Source: CAD feature listing. Evaluate the final solid. Frame: model axes, mm. A direction names the side the tool comes from. Give positions to 0.01 mm unless a question says otherwise; leave off trailing zeros. Loops run counter-clockwise (first coordinate to the right, second up) from the corner with the lowest first, then second, coordinate; pieces in that order, holes last. Notation, with made-up numbers: M 5,-1 L 64,-1 A6 ccw 64,6 Z; hole C 30,-17 d5. An arc over 180 degrees is marked long. Answer in a Markdown table with one row per item.
```python
from build123d import *

# Parameters (mm, degrees)
SKETCH_1_W          = 9
SKETCH_1_H          = 9
EXTRUDE_1_DEPTH     = 81.5
SKETCH_2_W          = 7
SKETCH_2_H          = 7
CUT_EXTRUDE_1_DEPTH = 101.5
SKETCH_3_R          = 3
SKETCH_3_R_2        = 1.5
CUT_EXTRUDE_2_DEPTH = 111.5
SKETCH_4_R          = 3
CUT_EXTRUDE_3_DEPTH = 1


with BuildPart() as part:
    # ｽｹｯﾁ1 → ﾎﾞｽ - 押し出し1 (new body)
    with BuildSketch(Plane.XY):
        Rectangle(SKETCH_1_W, SKETCH_1_H)
    extrude(amount=EXTRUDE_1_DEPTH)

    # ｽｹｯﾁ2 → ｶｯﾄ - 押し出し1 (cut)
    with BuildSketch(Plane.XY.offset(81.5)):
        Rectangle(SKETCH_2_W, SKETCH_2_H)
    extrude(amount=-CUT_EXTRUDE_1_DEPTH, mode=Mode.SUBTRACT)

    # ｽｹｯﾁ3 → ｶｯﾄ - 押し出し2 (cut)
    with BuildSketch(Plane(origin=(0, 4.5, 0), x_dir=(1, 0, 0), z_dir=(0, 1, 0))):
        with Locations((0, -5)):
            Circle(SKETCH_3_R)
        with Locations((0, -11.5)):
            Circle(SKETCH_3_R_2)
        with Locations((0, -76.5)):
            Circle(SKETCH_3_R_2)
    extrude(amount=-CUT_EXTRUDE_2_DEPTH, mode=Mode.SUBTRACT)

    # ｽｹｯﾁ4 → ｶｯﾄ - 押し出し3 (cut)
    with BuildSketch(Plane(origin=(0, 4.5, 0), x_dir=(1, 0, 0), z_dir=(0, 1, 0))):
        with Locations((0, -76.5)):
            Circle(SKETCH_4_R)
    extrude(amount=-CUT_EXTRUDE_3_DEPTH, mode=Mode.SUBTRACT)


solid = part.part
```
Q1. Section query D-D (z = 21). Output: boundary loops of the cut face in (x, y).
Values follow:
| item | result |
|---|---|
| outline | M -4.5,-4.5 L 4.5,-4.5 L 4.5,4.5 L -4.5,4.5 Z; hole M -3.5,-3.5 L 3.5,-3.5 L 3.5,3.5 L -3.5,3.5 Z |
Q2. Ray query, probe 1 along Z at (x, y) = (0, -4.05); probe 2 along X at (y, z) = (-4.1, 5); probe 3 along X at (y, z) = (2.5, 29.5). Return the intervals inside material, ascending. Write a range as from..to.
Values follow:
| item | result |
|---|---|
| probe 1 | 0..2, 8..10, 13..75, 78..81.5 |
| probe 2 | -4.5..-3, 3..4.5 |
| probe 3 | -4.5..-3.5, 3.5..4.5 |
Q3. Contact query for a flat-ended pin moving along its axis: pin 1 Ø1.8 at (x, z) = (0, 11.5) entering from -Y. Output: stop coordinate, or through.
Values follow:
| item | result |
|---|---|
| pin 1 | through |
Q4. Section query A-A (x = 0). Give the number of separate pieces and of enclosed holes in the cut face, plus the area to 3 significant figures.
Values follow:
| item | result |
|---|---|
| separate pieces | 8 |
| enclosed holes | 0 |
| area | 136 mm^2 |
Q5. Mould query, pull axis Z, two halves, no side actions, for faces 1 (the cylindrical face through (0, -4, 13)), 2 (the flat face through (-4, 0, 81.5)), 3 (the flat face through (0, 3.5, 41)). Classes: +Z half, -Z half, draft (parallel to the pull), parting line (faces both ways), or undercut.
Values follow:
| item | result |
|---|---|
| face 1 | undercut |
| face 2 | +Z half |
| face 3 | draft |
Q6. Section query B-B (z = 76.5). Output: boundary loops of the cut face in (x, y), plus the area to 3 significant figures.
Values follow:
| item | result |
|---|---|
| outline | M -4.5,-4.5 L -1.5,-4.5 L -1.5,-3.5 L -3.5,-3.5 L -3.5,3.5 L -3,3.5 L -3,4.5 L -4.5,4.5 Z; M 1.5,-4.5 L 4.5,-4.5 L 4.5,4.5 L 3,4.5 L 3,3.5 L 3.5,3.5 L 3.5,-3.5 L 1.5,-3.5 Z |
| area | 23.0 mm^2 |
Q7. Section query C-C (y = -2.5). Output: boundary loops of the cut face in (x, z), plus the area to 3 significant figures.
Values follow:
| item | result |
|---|---|
| outline | M -4.5,0 L -3.5,0 L -3.5,81.5 L -4.5,81.5 Z; M 3.5,0 L 4.5,0 L 4.5,81.5 L 3.5,81.5 Z |
| area | 163 mm^2 |
Q8. Reachability of faces 4 (the cylindrical face through (-0.65, 4.01, 79.43)), 5 (the cylindrical face through (0.806, -3.993, 75.235)), 6 (the flat face through (3.5, 0, 41)) from +Z, -Z, +X, -X, +Y, -Y: full face, straight path, thin tool, end or side. Return the list, or none.
Values follow:
| item | result |
|---|---|
| face 4 | +Y |
| face 5 | +Y, -Y |
| face 6 | +Z, -Z |
